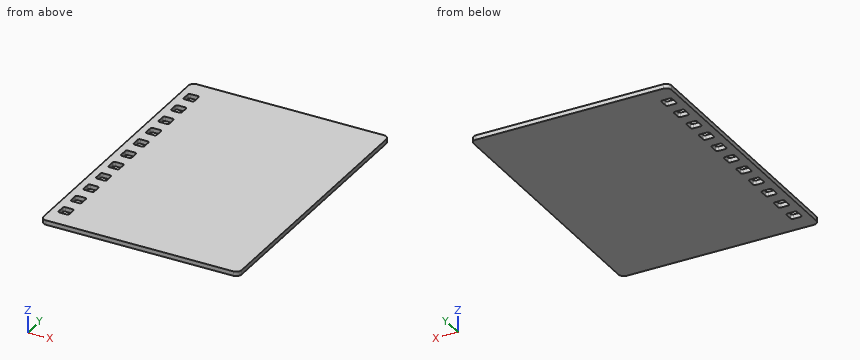
from build123d import *

# Parameters (mm, degrees)
BOSS_EXTRUDE1_DEPTH = 2.5


with BuildPart() as part:
    # Sketch1 → Boss-Extrude1 (new body)
    with BuildSketch(Plane.XY):
        with BuildLine():
            Line((3, 0), (108, 0))
            ThreePointArc((108, 0), (110.121320344, 0.878679656), (111, 3))
            Line((111, 3), (111, 151))
            ThreePointArc((111, 151), (110.121320344, 153.121320344), (108, 154))
            Line((108, 154), (3, 154))
            ThreePointArc((3, 154), (0.878679656, 153.121320344), (0, 151))
            Line((0, 151), (0, 3))
            ThreePointArc((0, 3), (0.878679656, 0.878679656), (3, 0))
        make_face()
        with BuildLine():
            Line((5, 22.8), (9, 22.8))
            ThreePointArc((9, 22.8), (9.707106781, 23.092893219), (10, 23.8))
            Line((10, 23.8), (10, 27.8))
            ThreePointArc((10, 27.8), (9.707106781, 28.507106781), (9, 28.8))
            Line((9, 28.8), (5, 28.8))
            ThreePointArc((5, 28.8), (4.292893219, 28.507106781), (4, 27.8))
            Line((4, 27.8), (4, 23.8))
            ThreePointArc((4, 23.8), (4.292893219, 23.092893219), (5, 22.8))
        make_face(mode=Mode.SUBTRACT)
        with BuildLine():
            Line((5, 16), (9, 16))
            ThreePointArc((9, 16), (9.707106781, 15.707106781), (10, 15))
            Line((10, 15), (10, 11))
            ThreePointArc((10, 11), (9.707106781, 10.292893219), (9, 10))
            Line((9, 10), (5, 10))
            ThreePointArc((5, 10), (4.292893219, 10.292893219), (4, 11))
            Line((4, 11), (4, 15))
            ThreePointArc((4, 15), (4.292893219, 15.707106781), (5, 16))
        make_face(mode=Mode.SUBTRACT)
        with BuildLine():
            Line((5, 35.6), (9, 35.6))
            ThreePointArc((9, 35.6), (9.707106781, 35.892893219), (10, 36.6))
            Line((10, 36.6), (10, 40.6))
            ThreePointArc((10, 40.6), (9.707106781, 41.307106781), (9, 41.6))
            Line((9, 41.6), (5, 41.6))
            ThreePointArc((5, 41.6), (4.292893219, 41.307106781), (4, 40.6))
            Line((4, 40.6), (4, 36.6))
            ThreePointArc((4, 36.6), (4.292893219, 35.892893219), (5, 35.6))
        make_face(mode=Mode.SUBTRACT)
        with BuildLine():
            Line((5, 48.4), (9, 48.4))
            ThreePointArc((9, 48.4), (9.707106781, 48.692893219), (10, 49.4))
            Line((10, 49.4), (10, 53.4))
            ThreePointArc((10, 53.4), (9.707106781, 54.107106781), (9, 54.4))
            Line((9, 54.4), (5, 54.4))
            ThreePointArc((5, 54.4), (4.292893219, 54.107106781), (4, 53.4))
            Line((4, 53.4), (4, 49.4))
            ThreePointArc((4, 49.4), (4.292893219, 48.692893219), (5, 48.4))
        make_face(mode=Mode.SUBTRACT)
        with BuildLine():
            Line((5, 61.2), (9, 61.2))
            ThreePointArc((9, 61.2), (9.707106781, 61.492893219), (10, 62.2))
            Line((10, 62.2), (10, 66.2))
            ThreePointArc((10, 66.2), (9.707106781, 66.907106781), (9, 67.2))
            Line((9, 67.2), (5, 67.2))
            ThreePointArc((5, 67.2), (4.292893219, 66.907106781), (4, 66.2))
            Line((4, 66.2), (4, 62.2))
            ThreePointArc((4, 62.2), (4.292893219, 61.492893219), (5, 61.2))
        make_face(mode=Mode.SUBTRACT)
        with BuildLine():
            Line((5, 74), (9, 74))
            ThreePointArc((9, 74), (9.707106781, 74.292893219), (10, 75))
            Line((10, 75), (10, 79))
            ThreePointArc((10, 79), (9.707106781, 79.707106781), (9, 80))
            Line((9, 80), (5, 80))
            ThreePointArc((5, 80), (4.292893219, 79.707106781), (4, 79))
            Line((4, 79), (4, 75))
            ThreePointArc((4, 75), (4.292893219, 74.292893219), (5, 74))
        make_face(mode=Mode.SUBTRACT)
        with BuildLine():
            Line((5, 86.8), (9, 86.8))
            ThreePointArc((9, 86.8), (9.707106781, 87.092893219), (10, 87.8))
            Line((10, 87.8), (10, 91.8))
            ThreePointArc((10, 91.8), (9.707106781, 92.507106781), (9, 92.8))
            Line((9, 92.8), (5, 92.8))
            ThreePointArc((5, 92.8), (4.292893219, 92.507106781), (4, 91.8))
            Line((4, 91.8), (4, 87.8))
            ThreePointArc((4, 87.8), (4.292893219, 87.092893219), (5, 86.8))
        make_face(mode=Mode.SUBTRACT)
        with BuildLine():
            Line((5, 99.6), (9, 99.6))
            ThreePointArc((9, 99.6), (9.707106781, 99.892893219), (10, 100.6))
            Line((10, 100.6), (10, 104.6))
            ThreePointArc((10, 104.6), (9.707106781, 105.307106781), (9, 105.6))
            Line((9, 105.6), (5, 105.6))
            ThreePointArc((5, 105.6), (4.292893219, 105.307106781), (4, 104.6))
            Line((4, 104.6), (4, 100.6))
            ThreePointArc((4, 100.6), (4.292893219, 99.892893219), (5, 99.6))
        make_face(mode=Mode.SUBTRACT)
        with BuildLine():
            Line((5, 112.4), (9, 112.4))
            ThreePointArc((9, 112.4), (9.707106781, 112.692893219), (10, 113.4))
            Line((10, 113.4), (10, 117.4))
            ThreePointArc((10, 117.4), (9.707106781, 118.107106781), (9, 118.4))
            Line((9, 118.4), (5, 118.4))
            ThreePointArc((5, 118.4), (4.292893219, 118.107106781), (4, 117.4))
            Line((4, 117.4), (4, 113.4))
            ThreePointArc((4, 113.4), (4.292893219, 112.692893219), (5, 112.4))
        make_face(mode=Mode.SUBTRACT)
        with BuildLine():
            Line((5, 125.2), (9, 125.2))
            ThreePointArc((9, 125.2), (9.707106781, 125.492893219), (10, 126.2))
            Line((10, 126.2), (10, 130.2))
            ThreePointArc((10, 130.2), (9.707106781, 130.907106781), (9, 131.2))
            Line((9, 131.2), (5, 131.2))
            ThreePointArc((5, 131.2), (4.292893219, 130.907106781), (4, 130.2))
            Line((4, 130.2), (4, 126.2))
            ThreePointArc((4, 126.2), (4.292893219, 125.492893219), (5, 125.2))
        make_face(mode=Mode.SUBTRACT)
        with BuildLine():
            Line((5, 138), (9, 138))
            ThreePointArc((9, 138), (9.707106781, 138.292893219), (10, 139))
            Line((10, 139), (10, 143))
            ThreePointArc((10, 143), (9.707106781, 143.707106781), (9, 144))
            Line((9, 144), (5, 144))
            ThreePointArc((5, 144), (4.292893219, 143.707106781), (4, 143))
            Line((4, 143), (4, 139))
            ThreePointArc((4, 139), (4.292893219, 138.292893219), (5, 138))
        make_face(mode=Mode.SUBTRACT)
    extrude(amount=BOSS_EXTRUDE1_DEPTH)


solid = part.part
Read the model definition and answer for the solid it produces. Units are mm, in the model's axes. Round coordinates to 2 decimals unless told otherwise and drop trailing zeros. Use one line per item in the form item = value. Start each with the question number.
(1) Find the intervals of material crossed by line 1 along X through (y, z) = (89.5, 1.05); line 2 along X through (y, z) = (67, 1.5), in increasing order. Write a range as from..to.
(2) A flat-ended cylindrical pin translates along its axis: pin 1 Ø3 at (x, y) = (38.5, 44.5) entering from -Z. Find the tip coordinate at first contact, or state that the pin passes through.
(3) The part is cut by section A-A (z = 1.9). Count the separate pieces of the cut face and the enclosed holes in it, then the cut area to 3 significant figures.
Checked values:
q1.line_1 = 0..4, 10..111
q1.line_2 = 0..4.4, 9.6..111
q2.pin_1 = 0
q3.separate_pieces = 1
q3.enclosed_holes = 11
q3.area = 16,700 mm^2
